Drawing for the job (mm, zero at the part's lowest x, y, z). Coordinates: 2 decimals unless noted, no trailing zeros. Order: outer loops, then holes, each group sorted by start corner. A loop starts at its lowest first (then second) coordinate and runs counter-clockwise, first axis right, second up.
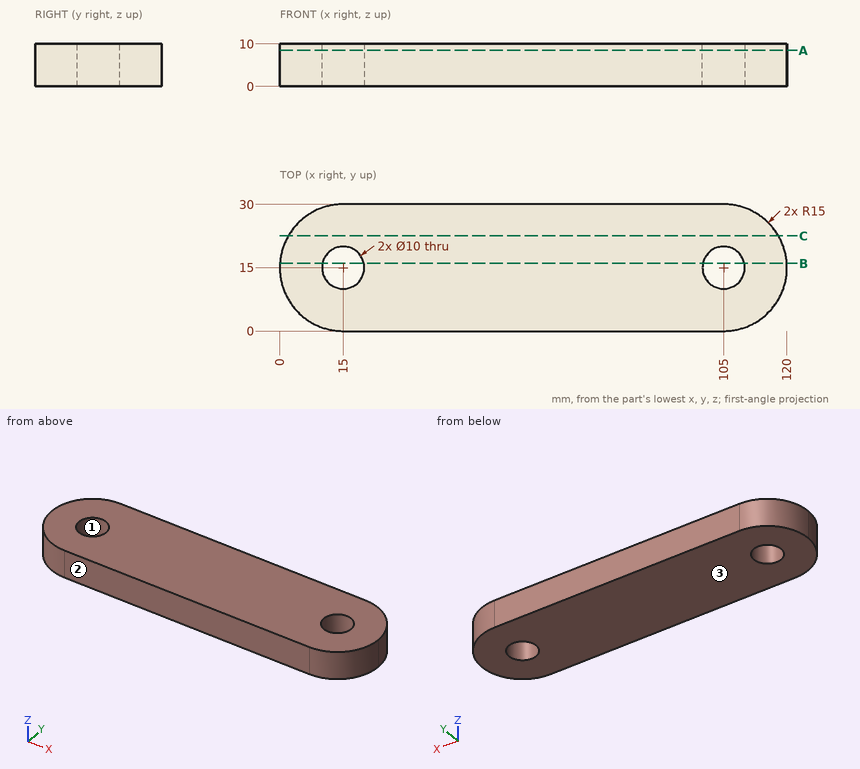
1) Slice it at A-A (z = 8.5). List the corners of the cut face in (x, y), plus the area to 3 significant figures.
2) Slice it at B-B (y = 16). List the corners of the cut face in (x, z).
3) Pin check, flat tip, straight feed: P1, Ø2, axis at x = 13.5, z = 9, coming from the -Y side. Stop position of the tip, or through.
4) Two-plate mould, pull along Y, no slides. Class the marked faces 1, 2 and 3: released by +Y, released by -Y, zero draft, split by the parting line, or undercut.
5) Slice it at C-C (y = 22.5). List the corners of the cut face in (x, z), plus the area to 3 significant figures.
6) Drill centre lines: probe 1 along X at (y, z) = (14, 1); probe 2 along Y at (x, z) = (108.5, 2.75); probe 3 along Y at (x, z) = (109, 7). Where is each one in solid material? Low to high.
Worked out:
1. outline: (0, 15) arc R15 ccw to (15, 0) - (105, 0) arc R15 ccw to (120, 15) arc R15 ccw to (105, 30) - (15, 30) arc R15 ccw to start; hole circle Ø10 at (15, 15); hole circle Ø10 at (105, 15)
1. area: 3,250 mm2
2. outline: (0.03, 0) - (10.1, 0) - (10.1, 10) - (0.03, 10) - close; (19.9, 0) - (100.1, 0) - (100.1, 10) - (19.9, 10) - close; (109.9, 0) - (119.97, 0) - (119.97, 10) - (109.9, 10) - close
3. P1: stops at y = 0.01
4. face 1: undercut
4. face 2: released by -Y
4. face 3: zero draft
5. outline: (2.01, 0) - (117.99, 0) - (117.99, 10) - (2.01, 10) - close
5. area: 1,160 mm2
6. probe 1: x = 0.03 to 10.1, 19.9 to 100.1, 109.9 to 119.97
6. probe 2: y = 0.41 to 11.43, 18.57 to 29.59
6. probe 3: y = 0.54 to 12, 18 to 29.46
